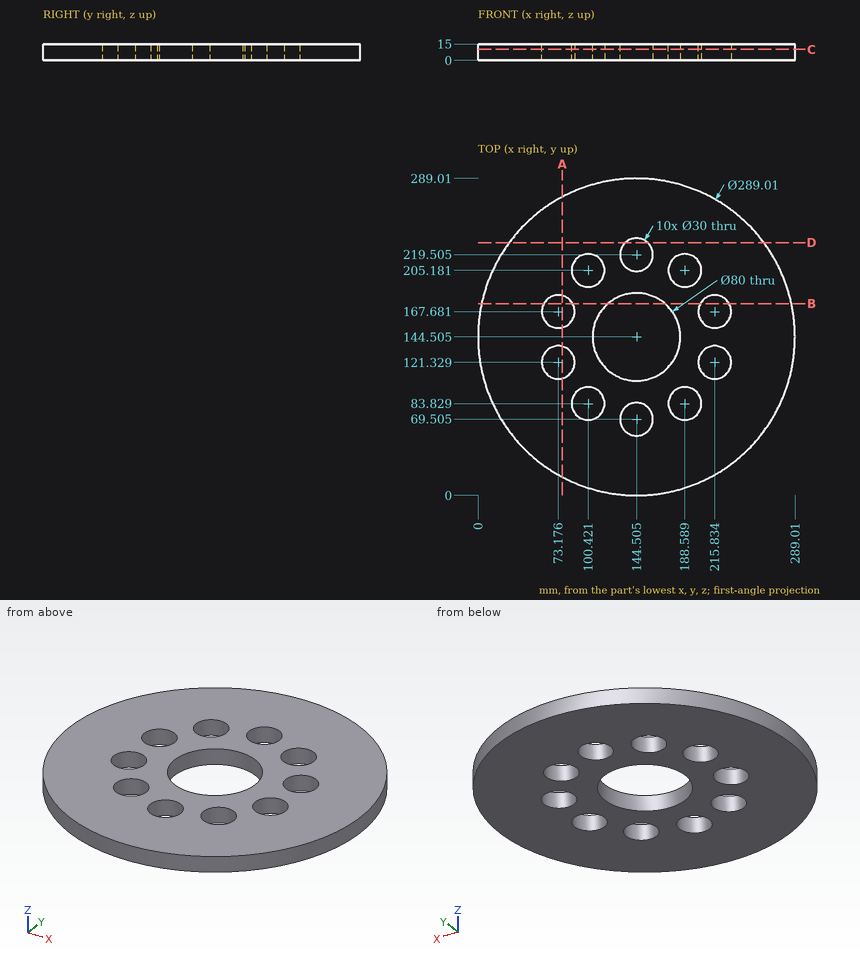
The drawing under review shows one solid part. Ordinate dimensions are in mm from its lowest x, y, z. Coordinates: 2 decimals unless noted, no trailing zeros. Order: outer loops, then holes, each group sorted by start corner. A loop starts at its lowest first (then second) coordinate and runs counter-clockwise, first axis right, second up. Notation, with made-up numbers: M 45,85.25 L 77,85.25 A26 cw 77,103.25 Z; hole C 85.25,-34.5 d2. An arc over 180 degrees is marked long. One line per question, with ' | ' between items.
(1) Add section C-C, the plane z = 10. State how many separate pieces and enclosed holes the cut face has, then the cut area to 3 significant figures.
Geometry results:
separate pieces: 1 | enclosed holes: 11 | area: 53,500 mm²
(2) Add section D-D, the plane y = 230.5. Write out the cut boundary in (x, z).
Geometry results:
outline: M 28.37,0 L 134.3,0 L 134.3,15 L 28.37,15 Z; M 154.71,0 L 260.64,0 L 260.64,15 L 154.71,15 Z
(3) Insertion check: pin 1 (1.5 mm diameter, centred on x = 112.5, z = 5, fed in from -Y); pin 2 (5 mm diameter, centred on y = 85.5, z = 13, fed in from -X) (1 decimal); pin 3 (1.5 mm diameter, centred on y = 183, z = 7, fed in from -X). Each pin has a flat end and moves straight along its axis. Give the tip position at first contact, or say it passes through.
Geometry results:
pin 1: stops at y = 3.42 | pin 2: stops at x = 11.5 | pin 3: stops at x = 5.02
(4) Add section B-B, the plane y = 175. Write out the cut boundary in (x, z), then the cut area to 3 significant figures.
Geometry results:
outline: M 3.25,0 L 60.08,0 L 60.08,15 L 3.25,15 Z; M 86.27,0 L 118.62,0 L 118.62,15 L 86.27,15 Z; M 170.39,0 L 202.74,0 L 202.74,15 L 170.39,15 Z; M 228.93,0 L 285.76,0 L 285.76,15 L 228.93,15 Z | area: 2,680 mm²
(5) Add section A-A, the plane x = 77. Write out the cut boundary in (y, z), then the cut area to 3 significant figures.
Geometry results:
outline: M 16.74,0 L 106.82,0 L 106.82,15 L 16.74,15 Z; M 135.83,0 L 153.18,0 L 153.18,15 L 135.83,15 Z; M 182.19,0 L 272.27,0 L 272.27,15 L 182.19,15 Z | area: 2,960 mm²
(6) For probe 1 along X at (y, z) = (128, 2.75) (1 decimal); probe 2 along X at (y, z) = (143.5, 5.5); probe 3 along X at (y, z) = (167.5, 4.5) (1 decimal), list the stretches that pass through material, from the lowest coordinate up. Write a range as from..to.
Geometry results:
probe 1: x = 0.9..59.7, 86.6..108.1, 180.9..202.4, 229.3..288.1 | probe 2: x = 0..104.52, 184.49..289.01 | probe 3: x = 1.8..58.2, 88.2..111.8, 177.2..200.8, 230.8..287.2
